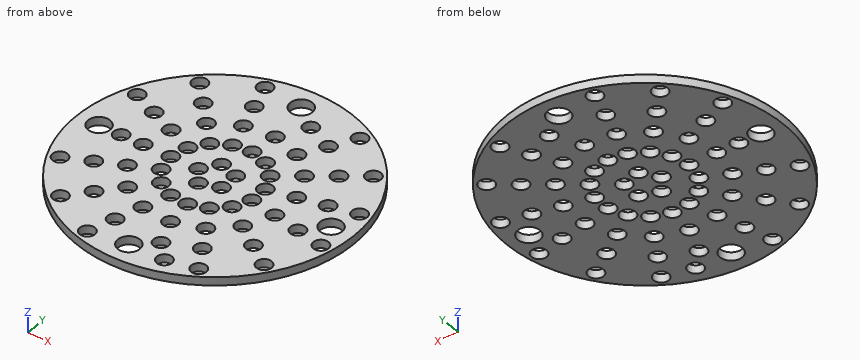
```python
from build123d import *

# Parameters (mm, degrees)
F0_R     = 50
F0_R_2   = 2.75
F0_R_3   = 4
F1_DEPTH = 3


with BuildPart() as f1:
    # F0 (on Top) → F1 (new body)
    with BuildSketch(Plane.XY):
        Circle(F0_R)
        with Locations((-30.221972, -34.678991)):
            Circle(F0_R_2, mode=Mode.SUBTRACT)
        with Locations((-13.558738, -43.956349)):
            Circle(F0_R_2, mode=Mode.SUBTRACT)
        with Locations((-23.651978, -27.14008)):
            Circle(F0_R_2, mode=Mode.SUBTRACT)
        with Locations((-10.611186, -34.400621)):
            Circle(F0_R_2, mode=Mode.SUBTRACT)
        with Locations((-41.690158, -19.44044)):
            Circle(F0_R_2, mode=Mode.SUBTRACT)
        with Locations((-32.62708, -15.214257)):
            Circle(F0_R_2, mode=Mode.SUBTRACT)
        with Locations((-17.081984, -19.601169)):
            Circle(F0_R_2, mode=Mode.SUBTRACT)
        with Locations((-7.663635, -24.844893)):
            Circle(F0_R_2, mode=Mode.SUBTRACT)
        with Locations((-4.716083, -15.289165)):
            Circle(F0_R_2, mode=Mode.SUBTRACT)
        with Locations((-23.564002, -10.988075)):
            Circle(F0_R_2, mode=Mode.SUBTRACT)
        with Locations((-14.500925, -6.761892)):
            Circle(F0_R_2, mode=Mode.SUBTRACT)
        with Locations((-10.51199, -12.062258)):
            Circle(F0_R_2, mode=Mode.SUBTRACT)
        with Locations((-1.768531, -5.733437)):
            Circle(F0_R_2, mode=Mode.SUBTRACT)
        with Locations((0, -42)):
            Circle(F0_R_3, mode=Mode.SUBTRACT)
        with Locations((12.873565, -42)):
            Circle(F0_R_2, mode=Mode.SUBTRACT)
        with Locations((23.494835, -39.547348)):
            Circle(F0_R_2, mode=Mode.SUBTRACT)
        with Locations((7.00363, -35.747819)):
            Circle(F0_R_2, mode=Mode.SUBTRACT)
        with Locations((3.072066, -25.81787)):
            Circle(F0_R_2, mode=Mode.SUBTRACT)
        with Locations((18.387262, -30.950098)):
            Circle(F0_R_2, mode=Mode.SUBTRACT)
        with Locations((37.5158, -26.61888)):
            Circle(F0_R_2, mode=Mode.SUBTRACT)
        with Locations((1.890502, -15.88792)):
            Circle(F0_R_2, mode=Mode.SUBTRACT)
        with Locations((8.172117, -13.755599)):
            Circle(F0_R_2, mode=Mode.SUBTRACT)
        with Locations((13.27969, -22.352849)):
            Circle(F0_R_2, mode=Mode.SUBTRACT)
        with Locations((21.204583, -15.045454)):
            Circle(F0_R_2, mode=Mode.SUBTRACT)
        with Locations((4.893365, -3.472028)):
            Circle(F0_R_2, mode=Mode.SUBTRACT)
        with Locations((13.048974, -9.258741)):
            Circle(F0_R_2, mode=Mode.SUBTRACT)
        with Locations((15.68276, -3.170338)):
            Circle(F0_R_2, mode=Mode.SUBTRACT)
        with Locations((29.360191, -20.832167)):
            Circle(F0_R_2, mode=Mode.SUBTRACT)
        with Locations((35.28621, -7.133261)):
            Circle(F0_R_2, mode=Mode.SUBTRACT)
        with Locations((25.484485, -5.1518)):
            Circle(F0_R_2, mode=Mode.SUBTRACT)
        with Locations((45.087934, -9.114723)):
            Circle(F0_R_2, mode=Mode.SUBTRACT)
        with Locations((-42, 0)):
            Circle(F0_R_3, mode=Mode.SUBTRACT)
        with Locations((-34, 0)):
            Circle(F0_R_2, mode=Mode.SUBTRACT)
        with Locations((-26, 0)):
            Circle(F0_R_2, mode=Mode.SUBTRACT)
        with Locations((-42.046383, 18.657482)):
            Circle(F0_R_2, mode=Mode.SUBTRACT)
        with Locations((-32.905865, 14.601508)):
            Circle(F0_R_2, mode=Mode.SUBTRACT)
        with Locations((-16, 0)):
            Circle(F0_R_2, mode=Mode.SUBTRACT)
        with Locations((-23.765347, 10.545534)):
            Circle(F0_R_2, mode=Mode.SUBTRACT)
        with Locations((-14.624829, 6.489559)):
            Circle(F0_R_2, mode=Mode.SUBTRACT)
        with Locations((-6, 0)):
            Circle(F0_R_2, mode=Mode.SUBTRACT)
        with Locations((-1.875431, 5.699365)):
            Circle(F0_R_2, mode=Mode.SUBTRACT)
        with Locations((-10.735703, 11.863586)):
            Circle(F0_R_2, mode=Mode.SUBTRACT)
        with Locations((-17.445517, 19.278328)):
            Circle(F0_R_2, mode=Mode.SUBTRACT)
        with Locations((-5.001148, 15.198306)):
            Circle(F0_R_2, mode=Mode.SUBTRACT)
        with Locations((-8.126866, 24.697248)):
            Circle(F0_R_2, mode=Mode.SUBTRACT)
        with Locations((-30.865146, 34.107811)):
            Circle(F0_R_2, mode=Mode.SUBTRACT)
        with Locations((-24.155331, 26.69307)):
            Circle(F0_R_2, mode=Mode.SUBTRACT)
        with Locations((-11.252584, 34.196189)):
            Circle(F0_R_2, mode=Mode.SUBTRACT)
        with Locations((-14.378301, 43.695131)):
            Circle(F0_R_2, mode=Mode.SUBTRACT)
        with Locations((4.827587, 3.562921)):
            Circle(F0_R_2, mode=Mode.SUBTRACT)
        with Locations((15.620736, 3.463034)):
            Circle(F0_R_2, mode=Mode.SUBTRACT)
        with Locations((12.873564, 9.501123)):
            Circle(F0_R_2, mode=Mode.SUBTRACT)
        with Locations((1.593086, 15.920492)):
            Circle(F0_R_2, mode=Mode.SUBTRACT)
        with Locations((7.913474, 13.906003)):
            Circle(F0_R_2, mode=Mode.SUBTRACT)
        with Locations((20.919542, 15.439325)):
            Circle(F0_R_2, mode=Mode.SUBTRACT)
        with Locations((12.859395, 22.597256)):
            Circle(F0_R_2, mode=Mode.SUBTRACT)
        with Locations((25.383696, 5.62743)):
            Circle(F0_R_2, mode=Mode.SUBTRACT)
        with Locations((35.146656, 7.791826)):
            Circle(F0_R_2, mode=Mode.SUBTRACT)
        with Locations((42, 0)):
            Circle(F0_R_3, mode=Mode.SUBTRACT)
        with Locations((44.909616, 9.956222)):
            Circle(F0_R_2, mode=Mode.SUBTRACT)
        with Locations((28.96552, 21.377527)):
            Circle(F0_R_2, mode=Mode.SUBTRACT)
        with Locations((2.588764, 25.8708)):
            Circle(F0_R_2, mode=Mode.SUBTRACT)
        with Locations((8.034443, 35.821106)):
            Circle(F0_R_2, mode=Mode.SUBTRACT)
        with Locations((17.805316, 31.288508)):
            Circle(F0_R_2, mode=Mode.SUBTRACT)
        with Locations((0, 42)):
            Circle(F0_R_3, mode=Mode.SUBTRACT)
        with Locations((22.751237, 39.97976)):
            Circle(F0_R_2, mode=Mode.SUBTRACT)
        with Locations((37.011498, 27.315729)):
            Circle(F0_R_2, mode=Mode.SUBTRACT)
    extrude(amount=F1_DEPTH)


solid = f1.part
```
Here's how the part is built. I have some questions about the finished solid (model axes, mm). Coordinates: 2 decimals unless noted, no trailing zeros. Order: outer loops, then holes, each group sorted by start corner. A loop starts at its lowest first (then second) coordinate and runs counter-clockwise, first axis right, second up.
Item 1: I'm going to push flat-ended pins straight in: pin 1 Ø3 at (x, y) = (7.5, -1.5) entering from -Z; pin 2 Ø1 at (x, z) = (-32, 0.5) entering from -Y. Where does each tip first touch, or does it pass through?
Response values:
pin 1: stops at z = 0
pin 2: stops at y = -38.83
Item 2: I need wall thicknesses on probe 1 along Y at (x, z) = (-41.5, 0.2); probe 2 along Y at (x, z) = (-24, 0.95); probe 3 along Y at (x, z) = (12, 2.5). Which ranges of each line are inside material? Lowest first, please.
Response values:
probe 1: y = -27.89 to -22.18, -16.7 to -3.97, 3.97 to 15.96, 21.35 to 27.89
probe 2: y = -43.86 to -29.87, -24.41 to -13.7, -8.27 to -1.89, 1.89 to 7.81, 13.29 to 23.95, 29.44 to 43.86
probe 3: y = -48.54 to -44.61, -39.39 to -24.79, -19.92 to -11.8, -6.72 to 6.89, 12.11 to 19.98, 25.21 to 48.54
Item 3: If we section it at B-B, the plane z = 1.1: Give the number of separate pieces and of enclosed holes in the cut face, then the cut area to 3 significant figures.
Response values:
separate pieces: 1
enclosed holes: 67
area: 6,160 mm2
Item 4: If we section it at A-A, the plane x = -25: List the corners of the cut face in (y, z) for me, then the cut area to 3 significant figures.
Response values:
outline: (-43.3, 0) - (-29.54, 0) - (-29.54, 3) - (-43.3, 3) - close; (-24.74, 0) - (-13.33, 0) - (-13.33, 3) - (-24.74, 3) - close; (-8.64, 0) - (-2.56, 0) - (-2.56, 3) - (-8.64, 3) - close; (2.56, 0) - (8.09, 0) - (8.09, 3) - (2.56, 3) - close; (13, 0) - (24.08, 0) - (24.08, 3) - (13, 3) - close; (29.31, 0) - (43.3, 0) - (43.3, 3) - (29.31, 3) - close
area: 186 mm2
